Can you work these out from the model? Positions are in its coordinate system, mm. A direction names the side the tool comes from. Round coordinates to 2 decimals unless told otherwise and drop trailing zeros. Write each loop counter-clockwise with the first axis right and the second up, starting at its lowest first coordinate (ties: lowest second). Pieces come first, ordered by that corner, then holes. Notation, with made-up numbers: (48.25, 22.5) - (80.25, 22.5) arc R25 cw to (80.25, 61.5) - close; hole circle Ø8 at (-22, 89). An arc over 180 degrees is marked (long way). One line per item, written item: value. Start each with the question number.
(1) I want a section at B-B on z = 92. List the corners of the cut face in (x, y) for me.
(2) If I drill on L1, parallel to Y at x = 1.4, z = 45; L2, parallel to Y at x = 1.9, z = 10; L3, parallel to Z at x = 0.7, y = 26.5, over which ranges is the centre line in solid material (lowest first)? Write a range as from..to.
(3) I want a section at D-D on x = 1.6. Give the number of separate pieces and of enclosed holes in the cut face, plus the area to 3 significant figures.
(4) I want a section at A-A on z = 120. List the corners of the cut face in (x, y) for me, plus the area to 3 significant figures.
(5) I want a section at C-C on y = -10. List the corners of the cut face in (x, z) for me.
(6) Thinking about a two-plate mould opening in Z: for faces 5 (the face through (2, -28, -3.3)), 6 (the face through (3.2, -8, 64)), 7 (the face through (1.58, -13.91, 73.35)), which applies, +Z half, -Z half, draft (parallel to the pull), parting line (faces both ways), or undercut?
(7) I'm going to push flat-ended pins straight in: pin 1 Ø1.6 at (x, y) = (1, 29) entering from -Z; pin 2 Ø1 at (x, z) = (2, -1.5) entering from -Y; pin 3 Ø1 at (x, z) = (1, -2.5) entering from +Y. Where does each tip first touch, or does it pass through?
(8) On a 3-axis mill with a long thin cutter (end or side, diameter ignored), from which of +Z, -Z, +X, -X, +Y, -Y can I reach the whole of each face in a straight line? I mean faces 1 (the face through (2, -2, 0)), 2 (the face through (0, -8, 64)), 3 (the face through (2, -14, 40.4)), 4 (the face through (2, 10.244, -2)). Say none if no direction works.
from build123d import *

# Parameters (mm, degrees)
F0_R     = 1.6
F0_W     = 8
F0_H     = 3.3
F0_W_2   = 19
F0_H_2   = 19
F0_R_2   = 1.1
F1_DEPTH = 3.2


# Not quite as in the source:
# - a feature names something its author has since deleted; it is built from what else it names


with BuildPart() as f1:
    # F0 (on Right) → F1 (new body)
    with BuildSketch(Plane.YZ):
        with BuildLine():
            ThreePointArc((-16.7558317706, 130), (-29.483753832, 124.7279220614), (-34.7558317706, 112))
            Line((-34.7558317706, 112), (-34.7558317706, 0))
            Line((-34.7558317706, 0), (-31.7558317706, 0))
            Line((-31.7558317706, 0), (-23.7558317706, 0))
            Line((-23.7558317706, 0), (-14.7558317706, 0))
            Line((-14.7558317706, 0), (-6.7558317706, 0))
            Line((-6.7558317706, 0), (2.2441682294, 0))
            Line((2.2441682294, 0), (10.2441682294, 0))
            Line((10.2441682294, 0), (15.2441682294, 0))
            Line((15.2441682294, 0), (15.2441682294, 19.74954395))
            Line((15.2441682294, 19.74954395), (15.2441682294, 38.74954395))
            Line((15.2441682294, 38.74954395), (15.2441682294, 112))
            ThreePointArc((15.2441682294, 112), (9.9720902908, 124.7279220614), (-2.7558317706, 130))
            Line((-2.7558317706, 130), (-16.7558317706, 130))
        make_face()
        Polygon((-24.7558317706, 40.4), (-24.7558317706, 105.4), (-16.7558317706, 105.4), (5.2441682294, 105.4), (5.2441682294, 40.4), (-2.7558317706, 40.4), align=None, mode=Mode.SUBTRACT)
        with Locations((-9.7558317706, 120)):
            Circle(F0_R, mode=Mode.SUBTRACT)
        with Locations((-27.7558317706, -1.65)):
            Rectangle(F0_W, F0_H)
        with Locations((-10.7558317706, -1.65)):
            Rectangle(F0_W, F0_H)
        with Locations((24.7441682294, 29.24954395)):
            Rectangle(F0_W_2, F0_H_2)
        with Locations((24.7441682294, 29.24954395)):
            Circle(F0_R_2, mode=Mode.SUBTRACT)
        with Locations((6.2441682294, -1.65)):
            Rectangle(F0_W, F0_H)
        Polygon((-16.7558317706, 105.4), (-24.7558317706, 105.4), (-2.7558317706, 40.4), (5.2441682294, 40.4), align=None)
    extrude(amount=F1_DEPTH)


solid = f1.part
Established:
1. outline: (0, -34.76) - (3.2, -34.76) - (3.2, -24.76) - (0, -24.76) - close; (0, -20.22) - (3.2, -20.22) - (3.2, -12.22) - (0, -12.22) - close; (0, 5.24) - (3.2, 5.24) - (3.2, 15.24) - (0, 15.24) - close
2. L1: -34.76..-24.76, -4.31..3.69, 5.24..15.24
2. L2: -34.76..15.24
2. L3: 19.75..38.75
3. separate pieces: 1
3. enclosed holes: 4
3. area: 5,360 mm2
4. outline: (0, -32.88) - (3.2, -32.88) - (3.2, -11.36) - (0, -11.36) - close; (0, -8.16) - (3.2, -8.16) - (3.2, 13.37) - (0, 13.37) - close
4. area: 138 mm2
5. outline: (0, -3.3) - (3.2, -3.3) - (3.2, 40.4) - (0, 40.4) - close; (0, 61.8) - (3.2, 61.8) - (3.2, 85.44) - (0, 85.44) - close; (0, 105.4) - (3.2, 105.4) - (3.2, 118.42) - (0, 118.42) - close; (0, 121.58) - (3.2, 121.58) - (3.2, 130) - (0, 130) - close
6. face 5: -Z half
6. face 6: draft
6. face 7: undercut
7. pin 1: z = 19.75
7. pin 2: y = -31.76
7. pin 3: y = 10.24
8. face 1: -Z, +X, -X
8. face 2: +Z, -Z, -X, +Y, -Y
8. face 3: +X, -X
8. face 4: -Z, +X, -X, +Y
